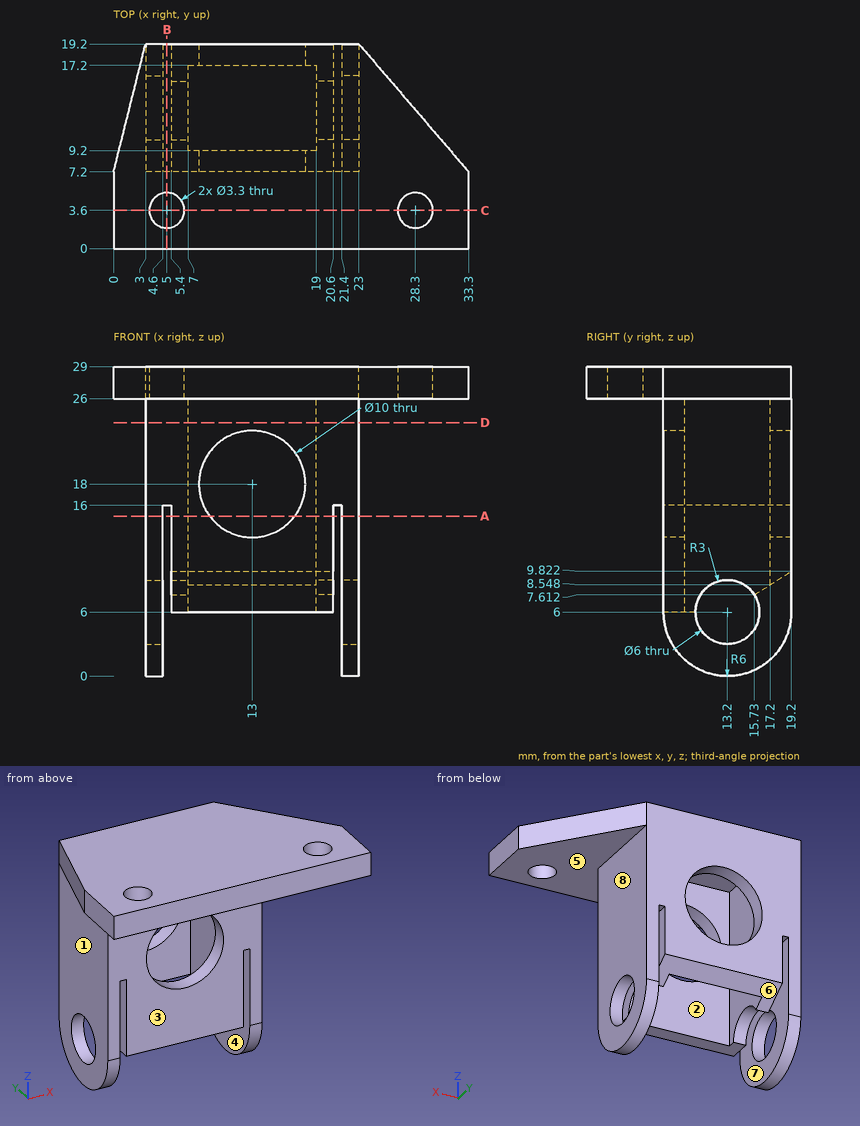
Source: three-view drawing plus pictorial views. Frame: mm from the lowest corner of the part. A direction names the side the tool comes from. Coordinates: 2 decimals unless noted, no trailing zeros. Order: outer loops, then holes, each group sorted by start corner. A loop starts at its lowest first (then second) coordinate and runs counter-clockwise, first axis right, second up. Notation, with made-up numbers: M 87,-16 L 98,-16 A13 ccw 98,-12 Z; hole C 70,79.25 d6. An arc over 180 degrees is marked long. Write each question's results on one line, items separated by ' | '. Start each with the question number.
1. Draft query along X for the marked faces 5, 6, 7 and 8. Return one class per face: +X half, -X half, draft (parallel to the pull), parting line (faces both ways), or undercut.
2. Section A-A, the plane z = 15. Return the cut outline in (x, y).
3. Section D-D, the plane z = 23.75. Return the cut outline in (x, y), then the cut area to 3 significant figures.
4. Section C-C, the plane y = 3.6. Return the cut outline in (x, z).
5. Reachability of the marked faces 1, 2, 3 and 4 from +Z, -Z, +X, -X, +Y, -Y: full face, straight path, thin tool, end or side. Return the list, or none.
6. Material intervals for L1, parallel to X at y = 12.5, z = 10.5; L2, parallel to Y at x = 22.45, z = 6; L3, parallel to Y at x = 5, z = 26.9, sorted ascending.
7. Pin query (flat end, axial travel): pin 1 (5 mm diameter, centred on y = 13.5, z = 11.5, fed in from -X); pin 2 (8 mm diameter, centred on x = 22.5, z = 13, fed in from -Y); pin 3 (9 mm diameter, centred on x = 15.5, y = 12, fed in from -Z). Return the tip coordinate at first contact, or that it passes through.
8. Section B-B, the plane x = 5. Return the cut outline in (y, z).
Solution:
1) face 5: draft | face 6: undercut | face 7: undercut | face 8: +X half
2) outline: M 3,7.2 L 4.6,7.2 L 4.6,19.2 L 3,19.2 Z; M 5.4,7.2 L 9,7.2 L 9,9.2 L 7,9.2 L 7,17.2 L 9,17.2 L 9,19.2 L 5.4,19.2 Z; M 17,7.2 L 20.6,7.2 L 20.6,19.2 L 17,19.2 L 17,17.2 L 19,17.2 L 19,9.2 L 17,9.2 Z; M 21.4,7.2 L 23,7.2 L 23,19.2 L 21.4,19.2 Z
3) outline: M 3,7.2 L 23,7.2 L 23,19.2 L 3,19.2 Z; hole M 7,9.2 L 19,9.2 L 19,17.2 L 7,17.2 Z | area: 144 mm²
4) outline: M 0,26 L 3.35,26 L 3.35,29 L 0,29 Z; M 6.65,26 L 26.65,26 L 26.65,29 L 6.65,29 Z; M 29.95,26 L 33.3,26 L 33.3,29 L 29.95,29 Z
5) face 1: -Z, -X, +Y, -Y | face 2: -Z | face 3: -Z, +X, -X, -Y | face 4: -Z, +Y, -Y
6) L1: 3 to 4.6, 5.4 to 7, 19 to 20.6, 21.4 to 23 | L2: 7.2 to 10.2, 16.2 to 19.2 | L3: 0 to 1.95, 5.25 to 19.2
7) pin 1: x = 3 | pin 2: y = 7.2 | pin 3: z = 6
8) outline: M 0,26 L 1.95,26 L 1.95,29 L 0,29 Z; M 5.25,26 L 7.2,26 L 7.2,16 L 19.2,16 L 19.2,29 L 5.25,29 Z
